The model under review builds one solid part; all positions refer to its coordinate system, in mm. A direction names the side the tool comes from. Coordinates: 2 decimals unless noted, no trailing zeros. Loops run counter-clockwise (first coordinate to the right, second up) from the corner with the lowest first, then second, coordinate; pieces in that order, holes last. Notation, with made-up numbers: (-30.5, 76.25) - (27.5, 76.25) arc R21 ccw to (27.5, 86.25) - close; hole circle Ø11 at (60, 26.25). An arc over 180 degrees is marked (long way). Use a Markdown table: item, result. Add a question column.
1) To check wall thickness, follow L1, parallel to X at y = 0.6, z = 0; L2, parallel to X at y = 2.2, z = 0; L3, parallel to X at y = 4.05, z = -2.25. State the ranges of each line that lie inside material, in increasing order. Write a range as [from, to].
2) For faces 1 (the flat face through (-2, 0, 0)), 2 (the cylindrical face through (1.352, 3.479, 4.292)), list the 3-axis set-ups (+Z, -Z, +X, -X, +Y, -Y) from which the entire face can be reached by the end or side of a thin tool; tool diameter is ignored.
3) The part is to be moulded in two halves that separate along X. For faces 3 (the flat face through (-4, 5, 0)), 4 (the cylindrical face through (-9.76, 0.99, -2.17)), 5 (the cylindrical face through (0.9, 2.77, 2.86)), say which applies: pulls with the +X half, pulls with the -X half, needs draft (parallel to the pull), parting line crosses it, or undercut.
4) Add section D-D, the plane y = 0.45. Give the boundary of the cut face in (x, z), and give its area (3 significant figures).
5) Clearance check with flat-ended pins moving along their axes: pin 1 (4 mm diameter, centred on x = 7, z = 0, fed in from +Y); pin 2 (2 mm diameter, centred on x = 5.5, y = 2, fed in from -Z); pin 3 (2 mm diameter, centred on x = -0.5, y = 3.5, fed in from +Z). State where each tip first meets the part, or that it passes through.
6) Add section C-C, the plane x = 7.75. Give the boundary of the cut face in (y, z).
7) Add section A-A, the plane x = 0. Give the boundary of the cut face in (y, z), and give its area (4 significant figures).
8) Add section B-B, the plane z = 0. Give the boundary of the cut face in (x, y).
```python
from build123d import *

# Parameters (mm, degrees)
SKETCH_1_R          = 10
EXTRUDE_1_DEPTH     = 2
SKETCH_2_R          = 4.5
EXTRUDE_2_DEPTH     = 3
SKETCH_3_R          = 1.5
CUT_EXTRUDE_1_DEPTH = 3
SKETCH_4_R          = 3
CUT_EXTRUDE_2_DEPTH = 4
SKETCH_5_R          = 1.5
CUT_EXTRUDE_3_DEPTH = 4
CHAMFER_2_SIZE      = 0.5


with BuildPart() as part:
    # 草图1 → 凸台-拉伸1 (new body)
    with BuildSketch(Plane(origin=(0, 0, 0), x_dir=(1, 0, 0), z_dir=(0, 1, 0))):
        with Locations(Location((0, 0, 0), (0, 0, 270))):
            Circle(SKETCH_1_R)
    extrude(amount=EXTRUDE_1_DEPTH)

    # 草图2 → 凸台-拉伸2 (add)
    with BuildSketch(Plane(origin=(0, 2, 0), x_dir=(1, 0, 0), z_dir=(0, 1, 0))):
        with Locations(Location((0, 0, 0), (0, 0, 270))):
            Circle(SKETCH_2_R)
    extrude(amount=EXTRUDE_2_DEPTH)

    # 草图3 → 切除-拉伸1 (cut)
    with BuildSketch(Plane(origin=(0, 2, 0), x_dir=(1, 0, 0), z_dir=(0, 1, 0))):
        with Locations(Location((-7, 0, 0), (0, 0, 270))):
            Circle(SKETCH_3_R)
        with Locations(Location((0, 7, 0), (0, 0, 270))):
            Circle(SKETCH_3_R)
        with Locations(Location((7, 0, 0), (0, 0, 270))):
            Circle(SKETCH_3_R)
        with Locations(Location((0, -7, 0), (0, 0, 270))):
            Circle(SKETCH_3_R)
    extrude(amount=-CUT_EXTRUDE_1_DEPTH, mode=Mode.SUBTRACT)

    # 草图4 → 切除-拉伸2 (cut)
    with BuildSketch(Plane(origin=(0, 5, 0), x_dir=(1, 0, 0), z_dir=(0, 1, 0))):
        with Locations(Location((0, 0, 0), (0, 0, 270))):
            Circle(SKETCH_4_R)
    extrude(amount=-CUT_EXTRUDE_2_DEPTH, mode=Mode.SUBTRACT)

    # 草图5 → 切除-拉伸3 (cut)
    with BuildSketch(Plane(origin=(0, 1, 0), x_dir=(1, 0, 0), z_dir=(0, 1, 0))):
        with Locations(Location((0, 0, 0), (0, 0, 270))):
            Circle(SKETCH_5_R)
    extrude(amount=-CUT_EXTRUDE_3_DEPTH, mode=Mode.SUBTRACT)

    # 倒角2
    chamfer_2_edges = [part.edges().sort_by_distance(p)[0] for p in [
        (0, 5, -3),
    ]]
    chamfer(chamfer_2_edges, length=CHAMFER_2_SIZE)


solid = part.part
```
From the geometry:
| question | item | result |
|---|---|---|
| 1 | L1 | x = [-10, -8.5], [-5.5, -1.5], [1.5, 5.5], [8.5, 10] |
| 1 | L2 | x = [-4.5, -3], [3, 4.5] |
| 1 | L3 | x = [-3.9, -1.98], [1.98, 3.9] |
| 2 | face 1 | +Z, -Z, +X, -X, -Y |
| 2 | face 2 | +Y |
| 3 | face 3 | needs draft |
| 3 | face 4 | parting line crosses it |
| 3 | face 5 | undercut |
| 4 | outline | circle Ø20 at (0, 0); hole circle Ø3 at (-7, 0); hole circle Ø3 at (0, -7); hole circle Ø3 at (0, 0); hole circle Ø3 at (0, 7); hole circle Ø3 at (7, 0) |
| 4 | area | 279 mm^2 |
| 5 | pin 1 | stops at y = 2 |
| 5 | pin 2 | stops at z = -8.93 |
| 5 | pin 3 | stops at z = 4.5 |
| 6 | outline | (0, -6.32) - (2, -6.32) - (2, -1.3) - (0, -1.3) - close; (0, 1.3) - (2, 1.3) - (2, 6.32) - (0, 6.32) - close |
| 7 | outline | (0, -10) - (2, -10) - (2, -8.5) - (0, -8.5) - close; (0, -5.5) - (2, -5.5) - (2, -4.5) - (5, -4.5) - (5, -3.5) - (4.5, -3) - (1, -3) - (1, -1.5) - (0, -1.5) - close; (0, 1.5) - (1, 1.5) - (1, 3) - (4.5, 3) - (5, 3.5) - (5, 4.5) - (2, 4.5) - (2, 5.5) - (0, 5.5) - close; (0, 8.5) - (2, 8.5) - (2, 10) - (0, 10) - close |
| 7 | area | 27.75 mm^2 |
| 8 | outline | (-10, 0) - (-8.5, 0) - (-8.5, 2) - (-10, 2) - close; (-5.5, 0) - (-1.5, 0) - (-1.5, 1) - (-3, 1) - (-3, 4.5) - (-3.5, 5) - (-4.5, 5) - (-4.5, 2) - (-5.5, 2) - close; (1.5, 0) - (5.5, 0) - (5.5, 2) - (4.5, 2) - (4.5, 5) - (3.5, 5) - (3, 4.5) - (3, 1) - (1.5, 1) - close; (8.5, 0) - (10, 0) - (10, 2) - (8.5, 2) - close |
